Verification items for the finished model (mm, model axes). A direction names the side the tool comes from. Give positions to 0.01 mm unless a question says otherwise; leave off trailing zeros. Order: outer loops, then holes, each group sorted by start corner. A loop starts at its lowest first (then second) coordinate and runs counter-clockwise, first axis right, second up. Notation, with made-up numbers: (40.5, 35.25) - (55.5, 35.25) arc R24 cw to (55.5, 63.25) - close; hole circle Ø3 at (-27.75, 42.25). An arc over 180 degrees is marked (long way). Answer as a JSON object with one key per item and string values.
```python
from build123d import *

# Parameters (mm, degrees)
F1_DEPTH = 124.46
F2_W     = 31.75
F2_H     = 24.671034
F3_DEPTH = 8.636
F4_W     = 18.288
F4_H     = 15.24
F5_DEPTH = 2.541


with BuildPart() as f1:
    # F0 (on Front) → F1 (new body)
    with BuildSketch(Plane.XZ):
        Polygon((-29.591, 0), (0, 0), (29.591, 0), (29.591, 11.738517), (27.772915, 13.512261), (25.999171, 11.694176), (27.051, 10.668), (27.051, 2.54), (0, 2.54), (-27.051, 2.54), (-27.051, 10.668), (-25.999171, 11.694176), (-27.772915, 13.512261), (-29.591, 11.738517), align=None)
    extrude(amount=F1_DEPTH)

    # F2 (on face) → F3 (cut)
    with BuildSketch(Plane.YZ.offset(29.591)):
        with Locations((-92.075, 14.875517)):
            Rectangle(F2_W, F2_H)
    extrude(amount=-F3_DEPTH, mode=Mode.SUBTRACT)

    # F4 (on face) → F5 (cut, through all)
    with BuildSketch(Plane.XY.offset(2.54)):
        with Locations((-15.621, -114.3)):
            Rectangle(F4_W, F4_H)
    extrude(amount=-F5_DEPTH, mode=Mode.SUBTRACT)


solid = f1.part
```
(1) Release check for a two-part mould opening along X. For faces 1 (the flat face through (0, 0, 2)), 2 (the flat face through (-16, -121.92, 1)), 3 (the flat face through (29.591, -48, 6)) record: pulls with the +X half, pulls with the -X half, needs draft (parallel to the pull), parting line crosses it, or undercut.
Computed values:
{"face 1": "needs draft", "face 2": "undercut", "face 3": "pulls with the +X half"}
(2) Section check C-C (y = -75). Record the cut outline in (x, z), then the cut area to 3 significant figures.
Computed values:
{"outline": "(-29.59, 0) - (29.59, 0) - (29.59, 11.74) - (27.77, 13.51) - (26, 11.69) - (27.05, 10.67) - (27.05, 2.54) - (-27.05, 2.54) - (-27.05, 10.67) - (-26, 11.69) - (-27.77, 13.51) - (-29.59, 11.74) - close", "area": "205 mm²"}
(3) Material ranges on line 1 along X through (y, z) = (-41, 8.75); line 2 along Z through (x, y) = (-10, -46); line 3 along X through (y, z) = (-107.5, 4.25), recorded low to high. Write a range as [from, to].
Computed values:
{"line 1": "x = [-29.59, -27.05], [27.05, 29.59]", "line 2": "z = [0, 2.54]", "line 3": "x = [-29.59, -27.05]"}
(4) Section check D-D (x = 6.5). Record the cut outline in (y, z).
Computed values:
{"outline": "(-124.46, 0) - (0, 0) - (0, 2.54) - (-124.46, 2.54) - close"}
(5) Gauge pin test, flat end, axial feed: pin 1 Ø5 at (x, y) = (18.5, -19.5) entering from +Z. Record the tip position at first contact, or that the pin passes through.
Computed values:
{"pin 1": "stops at z = 2.54"}
(6) Section check B-B (x = -16). Record the cut outline in (y, z), then the cut area to 3 significant figures.
Computed values:
{"outline": "(-124.46, 0) - (-121.92, 0) - (-121.92, 2.54) - (-124.46, 2.54) - close; (-106.68, 0) - (0, 0) - (0, 2.54) - (-106.68, 2.54) - close", "area": "277 mm²"}
(7) Access from +Z, -Z, +X, -X, +Y, -Y to the whole of each face (thin tool, end or side, straight path). Record for faces 4 (the flat face through (27.051, -116, 7)), 5 (the flat face through (28, -107.95, 8)), 6 (the flat face through (0, -124.46, 2)), 7 (the flat face through (-6.477, -114, 1)).
Computed values:
{"face 4": "+Y, -Y", "face 5": "+Z, +X", "face 6": "+Z, -Z, +X, -X, -Y", "face 7": "+Z, -Z"}
(8) Section check A-A (z = 4.75). Record the cut outline in (x, y), then the cut area to 3 significant figures.
Computed values:
{"outline": "(-29.59, -124.46) - (-27.05, -124.46) - (-27.05, 0) - (-29.59, 0) - close; (27.05, -124.46) - (29.59, -124.46) - (29.59, -107.95) - (27.05, -107.95) - close; (27.05, -76.2) - (29.59, -76.2) - (29.59, 0) - (27.05, 0) - close", "area": "552 mm²"}
